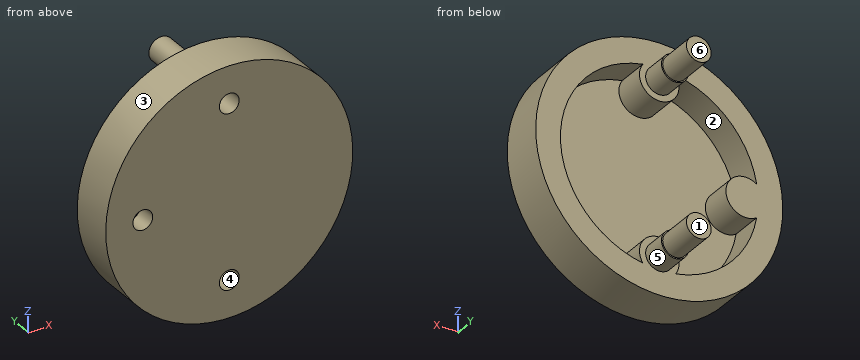
```python
from build123d import *

# Parameters (mm, degrees)
SKETCH1_R           = 50
BOSS_EXTRUDE1_DEPTH = 18
CUT_EXTRUDE1_START  = 5
SKETCH1_3_R         = 40
CUT_EXTRUDE1_DEPTH  = 13
BOSS_EXTRUDE2_REACH = 74.966
SKETCH2_R           = 8
SKETCH3_R           = 5.5
BOSS_EXTRUDE3_DEPTH = 10
SKETCH4_R           = 5
BOSS_EXTRUDE4_DEPTH = 15
SKETCH5_R           = 4
CUT_EXTRUDE2_DEPTH  = 18
SKETCH5_3_R         = 4
CUT_EXTRUDE3_DEPTH  = 8


with BuildPart() as part:
    # Sketch1 → Boss-Extrude1 (new body)
    with BuildSketch(Plane(origin=(0, 0, 0), x_dir=(1, 0, 0), z_dir=(0, 1, 0))):
        with Locations(Location((0, 0, 0), (0, 0, 270))):
            Circle(SKETCH1_R)
    extrude(amount=BOSS_EXTRUDE1_DEPTH)

    # Sketch1_3 → Cut-Extrude1 (cut)
    with BuildSketch(Plane(origin=(0, 0, 0), x_dir=(1, 0, 0), z_dir=(0, 1, 0)).offset(CUT_EXTRUDE1_START)):
        with Locations(Location((0, 0, 0), (0, 0, 90))):
            Circle(SKETCH1_3_R)
    extrude(amount=CUT_EXTRUDE1_DEPTH, mode=Mode.SUBTRACT)

    # Sketch2 → Boss-Extrude2 (add, up to next)
    with BuildSketch(Plane(origin=(0, 18, 0), x_dir=(1, 0, 0), z_dir=(0, 1, 0)), mode=Mode.PRIVATE) as boss_extrude2_sk1:
        with Locations((0, 35)):
            Circle(SKETCH2_R)
    boss_extrude2_tool1 = extrude(boss_extrude2_sk1.sketch, amount=-BOSS_EXTRUDE2_REACH, mode=Mode.PRIVATE) - part.part
    # Sketch2 → Boss-Extrude2 (add, up to next)
    with BuildSketch(Plane(origin=(0, 18, 0), x_dir=(1, 0, 0), z_dir=(0, 1, 0)), mode=Mode.PRIVATE) as boss_extrude2_sk2:
        with Locations((0, -35)):
            Circle(SKETCH2_R)
    boss_extrude2_tool2 = extrude(boss_extrude2_sk2.sketch, amount=-BOSS_EXTRUDE2_REACH, mode=Mode.PRIVATE) - part.part
    # Sketch2 → Boss-Extrude2 (add, up to next)
    with BuildSketch(Plane(origin=(0, 18, 0), x_dir=(1, 0, 0), z_dir=(0, 1, 0)), mode=Mode.PRIVATE) as boss_extrude2_sk3:
        with Locations((-35, 0)):
            Circle(SKETCH2_R)
    boss_extrude2_tool3 = extrude(boss_extrude2_sk3.sketch, amount=-BOSS_EXTRUDE2_REACH, mode=Mode.PRIVATE) - part.part
    add(boss_extrude2_tool1.solids().sort_by_distance((0, 18, -35))[0])
    add(boss_extrude2_tool2.solids().sort_by_distance((0, 18, 35))[0])
    add(boss_extrude2_tool3.solids().sort_by_distance((-35, 18, 0))[0])

    # Sketch3 → Boss-Extrude3 (add)
    with BuildSketch(Plane(origin=(0, 18, 0), x_dir=(1, 0, 0), z_dir=(0, 1, 0))):
        with Locations(Location((0, 35, 0), (0, 0, 270))):
            Circle(SKETCH3_R)
        with Locations(Location((0, -35, 0), (0, 0, 270))):
            Circle(SKETCH3_R)
    extrude(amount=BOSS_EXTRUDE3_DEPTH)

    # Sketch4 → Boss-Extrude4 (add)
    with BuildSketch(Plane(origin=(0, 28, 0), x_dir=(1, 0, 0), z_dir=(0, 1, 0))):
        with Locations(Location((0, -35, 0), (0, 0, 270))):
            Circle(SKETCH4_R)
        with Locations(Location((0, 35, 0), (0, 0, 270))):
            Circle(SKETCH4_R)
    extrude(amount=BOSS_EXTRUDE4_DEPTH)

    # Sketch5 → Cut-Extrude2 (cut)
    with BuildSketch(Plane.XZ):
        with Locations(Location((0, 35, 0), (0, 0, 270))):
            Circle(SKETCH5_R)
        with Locations(Location((0, -35, 0), (0, 0, 270))):
            Circle(SKETCH5_R)
    extrude(amount=-CUT_EXTRUDE2_DEPTH, mode=Mode.SUBTRACT)

    # Sketch5_3 → Cut-Extrude3 (cut)
    with BuildSketch(Plane.XZ):
        with Locations(Location((-35, 0, 0), (0, 0, 270))):
            Circle(SKETCH5_3_R)
    extrude(amount=-CUT_EXTRUDE3_DEPTH, mode=Mode.SUBTRACT)


solid = part.part
```
Read the model definition and answer for the solid it produces. Units are mm, in the model's axes. Face numbers are marked on the shaded views. A direction names the side the tool comes from. Coordinates: 2 decimals unless noted, no trailing zeros. Write each loop counter-clockwise with the first axis right and the second up, starting at its lowest first coordinate (ties: lowest second). Pieces come first, ordered by that corner, then holes. Notation, with made-up numbers: (55, 9.5) - (92, 9.5) arc R23 ccw to (92, 39.5) - close; hole circle Ø4 at (30, 70.25). An arc over 180 degrees is marked (long way). Answer as a JSON object with one key per item and string values. Group by question number.
1. A cutting plane is placed at A-A (y = 13). Determine the outline of the cut face in (x, z).
2. Consider L1, parallel to X at y = 2, z = 0; L2, parallel to Z at x = -36.5, y = 7.5; L3, parallel to X at y = 14.5, z = 35. Determine where each line is inside the solid, lowest interval first. Write a range as [from, to].
3. A cutting plane is placed at C-C (z = 0). Determine the outline of the cut face in (x, y).
4. A cutting plane is placed at D-D (y = 24.5). Determine the outline of the cut face in (x, z), plus the area to 3 significant figures.
5. The mould has two halves that part along X. Classify the marked faces 1, 2 and 3: +X half, -X half, draft (parallel to the pull), parting line (faces both ways), or undercut.
6. Each of these flat-tipped pins is pushed along its axis until it touches: P1, Ø2.5, axis at x = 1, z = 33.5, coming from the -Y side; P2, Ø2, axis at x = -32, z = 34.5, coming from the +Y side; P3, Ø1.5, axis at y = 21, z = 39, coming from the -X side. Where does it stop, or does it pass through?
7. Which of the six approach directions +Z, -Z, +X, -X, +Y, -Y give full straight-line access (tool end or side, diameter ignored) to the marked faces 4, 5 and 6?
Worked out:
{
 "1": {"outline": "circle Ø100 at (0, 0); hole (-39.44, -6.65) arc R40 ccw to (-6.65, -39.44) arc R8 cw (long way) to (6.65, -39.44) arc R40 ccw to (6.65, 39.44) arc R8 cw (long way) to (-6.65, 39.44) arc R40 ccw to (-39.44, 6.65) arc R8 cw (long way) to start; hole circle Ø8 at (0, -35); hole circle Ø8 at (0, 35)"},
 "2": {"L1": "x = [-50, -39], [-31, 50]", "L2": "z = [-34.17, -16.36], [-7.86, -3.71], [3.71, 7.86], [16.36, 34.17]", "L3": "x = [-35.71, -19.36], [-8, -4], [4, 8], [19.36, 35.71]"},
 "3": {"outline": "(-50, 0) - (-39, 0) - (-39, 8) - (-31, 8) - (-31, 0) - (50, 0) - (50, 18) - (40, 18) - (40, 5) - (-27, 5) - (-27, 18) - (-50, 18) - close"},
 "4": {"outline": "circle Ø11 at (0, -35); circle Ø11 at (0, 35)", "area": "190 mm²"},
 "5": {"face 1": "draft", "face 2": "undercut", "face 3": "parting line"},
 "6": {"P1": "stops at y = 18", "P2": "stops at y = 18", "P3": "stops at x = -4.44"},
 "7": {"face 4": "-Y", "face 5": "+Y", "face 6": "+Z, -Z, +X, -X, +Y"}
}
